Job drawing, mm, ordinate dimensions from the low corner. One solid piece. Coordinates: 2 decimals unless noted, no trailing zeros. Order: outer loops, then holes, each group sorted by start corner. A loop starts at its lowest first (then second) coordinate and runs counter-clockwise, first axis right, second up. Notation, with made-up numbers: (-7, 35) - (2, 35) arc R16 ccw to (2, 51) - close; hole circle Ø10 at (0.25, -3.5). An arc over 180 degrees is marked (long way). Write each question's results on one line, items separated by ' | '. Start each with the question number.
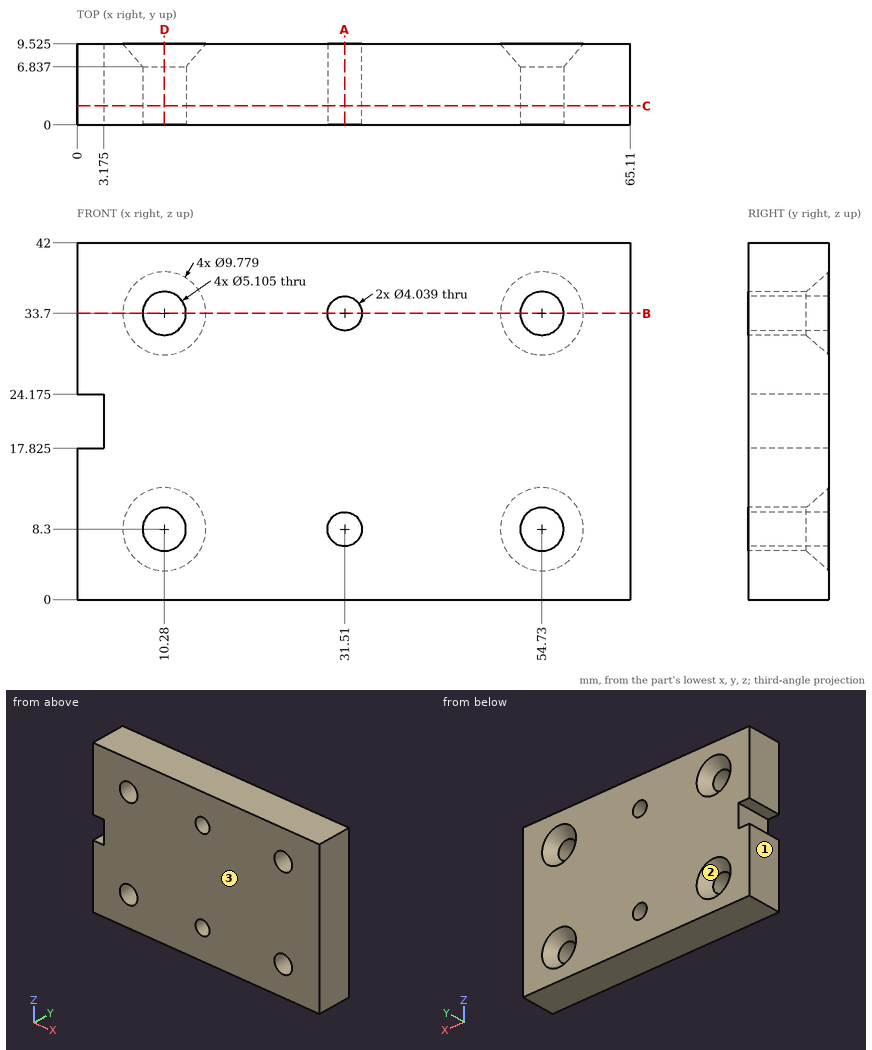
Item 1: Slice it at A-A (x = 31.51). Write the cut outline in (y, z) (1 decimal).
Item 2: Slice it at C-C (y = 2.25). Write the cut outline in (x, z) (1 decimal), then the cut area to 3 significant figures.
Item 3: Pull direction X, two halves, no side cores. Call the marked faces 1, 2 and 3: released by +X, released by -X, zero draft, split by the parting line, or undercut.
Item 4: Probe probe 1 along Z at (x, y) = (10.28, 5.25); probe 2 along X at (y, z) = (2.75, 8.3); probe 3 along Z at (x, y) = (31.51, 5). List the from-to ranges inside material, lowest first.
Item 5: Flat gauge pin, fed straight in: P1, Ø3, axis at y = 5.5, z = 20.5, coming from the -X side (3 decimals). Where does the tip first touch, or does it go through?
Item 6: Slice it at B-B (z = 33.7). Write the cut outline in (x, y) (1 decimal).
Item 7: Slice it at D-D (x = 10.28). Write the cut outline in (y, z) (1 decimal), then the cut area to 3 significant figures.
Resolved:
1) outline: (0, 0) - (9.5, 0) - (9.5, 6.3) - (0, 6.3) - close; (0, 10.3) - (9.5, 10.3) - (9.5, 31.7) - (0, 31.7) - close; (0, 35.7) - (9.5, 35.7) - (9.5, 42) - (0, 42) - close
2) outline: (0, 0) - (65.1, 0) - (65.1, 42) - (0, 42) - (0, 24.2) - (3.2, 24.2) - (3.2, 17.8) - (0, 17.8) - close; hole circle Ø5.1 at (10.3, 8.3); hole circle Ø5.1 at (10.3, 33.7); hole circle Ø4 at (31.5, 8.3); hole circle Ø4 at (31.5, 33.7); hole circle Ø5.1 at (54.7, 8.3); hole circle Ø5.1 at (54.7, 33.7) | area: 2,610 mm^2
3) face 1: released by -X | face 2: undercut | face 3: zero draft
4) probe 1: 0 to 5.75, 10.85 to 31.15, 36.25 to 42 | probe 2: 0 to 7.73, 12.83 to 29.49, 33.53 to 52.18, 57.28 to 65.11 | probe 3: 0 to 6.28, 10.32 to 31.68, 35.72 to 42
5) P1: x = 3.175
6) outline: (0, 0) - (7.7, 0) - (7.7, 6.8) - (5.4, 9.5) - (0, 9.5) - close; (12.8, 0) - (29.5, 0) - (29.5, 9.5) - (15.2, 9.5) - (12.8, 6.8) - close; (33.5, 0) - (52.2, 0) - (52.2, 6.8) - (49.8, 9.5) - (33.5, 9.5) - close; (57.3, 0) - (65.1, 0) - (65.1, 9.5) - (59.6, 9.5) - (57.3, 6.8) - close
7) outline: (0, 0) - (9.5, 0) - (9.5, 3.4) - (6.8, 5.7) - (0, 5.7) - close; (0, 10.9) - (6.8, 10.9) - (9.5, 13.2) - (9.5, 28.8) - (6.8, 31.1) - (0, 31.1) - close; (0, 36.3) - (6.8, 36.3) - (9.5, 38.6) - (9.5, 42) - (0, 42) - close | area: 290 mm^2
